Geometry check sheet. Reference: the model listing, model coordinates, mm. Face numbers are marked on the shaded views. Round coordinates to 2 decimals unless told otherwise and drop trailing zeros. Order: outer loops, then holes, each group sorted by start corner. A loop starts at its lowest first (then second) coordinate and runs counter-clockwise, first axis right, second up. Notation, with made-up numbers: (43.5, 8) - (92.5, 8) arc R20 ccw to (92.5, 41) - close; hole circle Ø5 at (52, 6.5). An arc over 180 degrees is marked (long way). One line per question, with ' | ' between items. Start each with the question number.
Q1. Sectioned sample at B-B, the plane x = 7.25. Enter the section's corners in (y, z), then the cut area to 3 significant figures.
Q2. Material ranges on line 1 along Y through (x, z) = (13.75, 0); line 2 along X through (y, z) = (2, 18.5); line 3 along Z through (x, y) = (7.75, -1), recorded low to high.
Q3. Mould release check, pull along Y, two halves, no side actions. Record for the marked faces 1, 2, 3 and 4: +Y half, -Y half, draft (parallel to the pull), parting line (faces both ways), or undercut.
Q4. Sectioned sample at D-D, the plane y = 14.5. Enter the section's corners in (x, z), then the cut area to 3 significant figures.
Q5. Sectioned sample at A-A, the plane z = 0. Enter the section's corners in (x, y), then the cut area to 3 significant figures.
Q6. Gauge pin test, flat ends, axial feed: P1, Ø5, axis at y = 0, z = -24, coming from the -X side; P2, Ø1.5, axis at x = 11, z = -6.5, coming from the -Y side; P3, Ø8, axis at y = 0, z = 24, coming from the +X side; P4, Ø5, axis at x = 6, y = 9.5, coming from the -Z side. Record the tip position at first contact, or that the pin passes through.
Q7. Sectioned sample at C-C, the plane y = 6.5. Enter the section's corners in (x, z), then the cut area to 3 significant figures.
```python
from build123d import *

# Parameters (mm, degrees)
SKETCH1_R           = 10
SKETCH1_R_2         = 3
BOSS_EXTRUDE1_DEPTH = 8
SKETCH3_R           = 17
SKETCH3_R_2         = 10
BOSS_EXTRUDE2_DEPTH = 20
FILLET1_R           = 5


with BuildPart() as part:
    # Sketch1 → Boss-Extrude1 (new body)
    with BuildSketch(Plane(origin=(0, 0, 0), x_dir=(0, 0, -1), z_dir=(1, 0, 0))):
        with BuildLine():
            Line((30, -6), (30, 6))
            Line((30, 6), (6.490927502, 15.712029155))
            ThreePointArc((6.490927502, 15.712029155), (0, 17), (-6.490927502, 15.712029155))
            Line((-6.490927502, 15.712029155), (-30, 6))
            Line((-30, 6), (-30, -6))
            Line((-30, -6), (-6.490927502, -15.712029155))
            ThreePointArc((-6.490927502, -15.712029155), (0, -17), (6.490927502, -15.712029155))
            Line((6.490927502, -15.712029155), (30, -6))
        make_face()
        Circle(SKETCH1_R, mode=Mode.SUBTRACT)
        with Locations((-24, 0)):
            Circle(SKETCH1_R_2, mode=Mode.SUBTRACT)
        with Locations((24, 0)):
            Circle(SKETCH1_R_2, mode=Mode.SUBTRACT)
    extrude(amount=BOSS_EXTRUDE1_DEPTH)

    # Sketch3 → Boss-Extrude2 (add)
    with BuildSketch(Plane(origin=(0, 0, 0), x_dir=(0, 0, -1), z_dir=(1, 0, 0))):
        Circle(SKETCH3_R)
        Circle(SKETCH3_R_2, mode=Mode.SUBTRACT)
    extrude(amount=BOSS_EXTRUDE2_DEPTH)

    # Fillet1
    fillet1_edges = [part.edges().sort_by_distance(p)[0] for p in [
        (4, 6, -30),
        (4, -6, -30),
        (4, -6, 30),
        (4, 6, 30),
    ]]
    fillet(fillet1_edges, radius=FILLET1_R)


solid = part.part
```
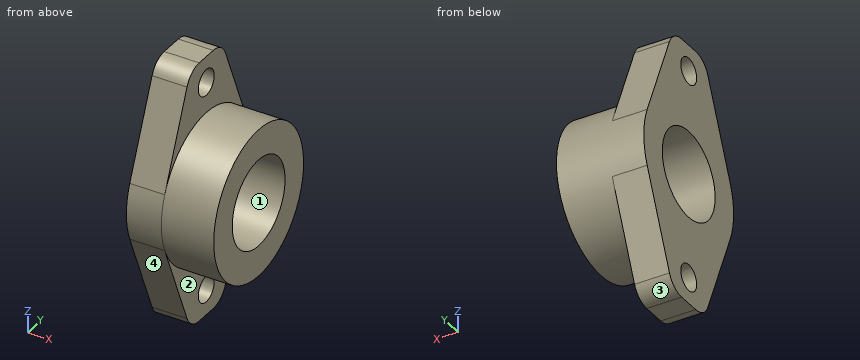
Determined:
1) outline: (-15.71, -6.49) - (-7.28, -26.91) arc R5 ccw to (-2.66, -30) - (2.66, -30) arc R5 ccw to (7.28, -26.91) - (15.71, -6.49) arc R17 ccw to (15.71, 6.49) - (7.28, 26.91) arc R5 ccw to (2.66, 30) - (-2.66, 30) arc R5 ccw to (-7.28, 26.91) - (-15.71, 6.49) arc R17 ccw to start; hole circle Ø20 at (0, 0); hole circle Ø6 at (0, -24); hole circle Ø6 at (0, 24) | area: 1,070 mm2
2) line 1: y = -17 to -10, 10 to 17 | line 2: x = 0 to 8 | line 3: z = -30 to -26.83, -21.17 to -9.95, 9.95 to 21.17, 26.83 to 30
3) face 1: undercut | face 2: draft | face 3: +Y half | face 4: -Y half
4) outline: (0, -9.42) - (8, -9.42) - (8, -8.87) - (20, -8.87) - (20, 8.87) - (8, 8.87) - (8, 9.42) - (0, 9.42) - close | area: 364 mm2
5) outline: (0, -17) - (20, -17) - (20, -10) - (0, -10) - close; (0, 10) - (20, 10) - (20, 17) - (0, 17) - close | area: 280 mm2
6) P1: passes through | P2: stops at y = -16 | P3: stops at x = 8 | P4: stops at z = -27.48
7) outline: (0, -28.2) - (8, -28.2) - (8, -15.71) - (20, -15.71) - (20, -7.6) - (0, -7.6) - close; (0, 7.6) - (20, 7.6) - (20, 15.71) - (8, 15.71) - (8, 28.2) - (0, 28.2) - close | area: 524 mm2
